```python
from build123d import *

# Parameters (mm, degrees)
EXTRUDE_1_DEPTH     = 20
SKETCH_9_W          = 35
SKETCH_9_H          = 3
EXTRUDE_2_DEPTH     = 5
SKETCH_10_W         = 3
SKETCH_10_H         = 35
EXTRUDE_3_DEPTH     = 5
SKETCH_11_R         = 8
CUT_EXTRUDE_4_DEPTH = 8
SKETCH_12_W         = 30
SKETCH_12_H         = 3
CUT_EXTRUDE_5_DEPTH = 18
SKETCH_13_W         = 30
SKETCH_13_H         = 17
CUT_EXTRUDE_6_DEPTH = 1
SKETCH_14_W         = 30
SKETCH_14_H         = 36
CUT_EXTRUDE_7_DEPTH = 1
SKETCH_15_R         = 1.5
CUT_EXTRUDE_8_DEPTH = 2
SKETCH_17_W         = 39.353314789
SKETCH_17_H         = 5.702998022
CUT_EXTRUDE_9_DEPTH = 8


with BuildPart() as part:
    # 草图1 → 凸台-拉伸1 (new body)
    with BuildSketch(Plane(origin=(0, 0, 0), x_dir=(0, 0, -1), z_dir=(1, 0, 0))):
        Polygon((0, 0), (0, 38), (3, 38), (3, 3), (38, 3), (38, 0), align=None)
    extrude(amount=EXTRUDE_1_DEPTH)

    # 草图9 → 凸台-拉伸2 (add)
    with BuildSketch(Plane(origin=(20, 0, 0), x_dir=(0, 0, -1), z_dir=(1, 0, 0))):
        Polygon((3, 38), (0, 38), (0, 0), (3, 0), (3, 3), align=None)
        with Locations((20.5, 1.5)):
            Rectangle(SKETCH_9_W, SKETCH_9_H)
    extrude(amount=EXTRUDE_2_DEPTH)

    # 草图10 → 凸台-拉伸3 (add)
    with BuildSketch(Plane.ZY):
        with Locations((-1.5, 20.5)):
            Rectangle(SKETCH_10_W, SKETCH_10_H)
        Polygon((0, 0), (0, 3), (-3, 3), (-38, 3), (-38, 0), align=None)
    extrude(amount=EXTRUDE_3_DEPTH)

    # 草图11 → 切除-拉伸4 (cut)
    with BuildSketch(Plane.XY):
        with Locations((10, 16)):
            Circle(SKETCH_11_R)
    extrude(amount=-CUT_EXTRUDE_4_DEPTH, mode=Mode.SUBTRACT)

    # 草图12 → 切除-拉伸5 (cut)
    with BuildSketch(Plane(origin=(0, 0, -38), x_dir=(-1, 0, 0), z_dir=(0, 0, -1))):
        with Locations((-10, 1.5)):
            Rectangle(SKETCH_12_W, SKETCH_12_H)
    extrude(amount=-CUT_EXTRUDE_5_DEPTH, mode=Mode.SUBTRACT)

    # 草图13 → 切除-拉伸6 (cut)
    with BuildSketch(Plane(origin=(0, 3, 0), x_dir=(1, 0, 0), z_dir=(0, 1, 0))):
        with Locations((10, 11.5)):
            Rectangle(SKETCH_13_W, SKETCH_13_H)
    extrude(amount=-CUT_EXTRUDE_6_DEPTH, mode=Mode.SUBTRACT)

    # 草图14 → 切除-拉伸7 (cut)
    with BuildSketch(Plane(origin=(0, 0, -3), x_dir=(-1, 0, 0), z_dir=(0, 0, -1))):
        with Locations((-10, 20)):
            Rectangle(SKETCH_14_W, SKETCH_14_H)
    extrude(amount=-CUT_EXTRUDE_7_DEPTH, mode=Mode.SUBTRACT)

    # 草图15 → 切除-拉伸8 (cut)
    with BuildSketch(Plane(origin=(0, 2, 0), x_dir=(1, 0, 0), z_dir=(0, 1, 0))):
        with Locations((20, 6)):
            Circle(SKETCH_15_R)
        with Locations((0, 6)):
            Circle(SKETCH_15_R)
        with Locations((0, 16)):
            Circle(SKETCH_15_R)
        with Locations((20, 16)):
            Circle(SKETCH_15_R)
    extrude(amount=-CUT_EXTRUDE_8_DEPTH, mode=Mode.SUBTRACT)

    # 草图17 → 切除-拉伸9 (cut)
    with BuildSketch(Plane(origin=(0, 38, 0), x_dir=(1, 0, 0), z_dir=(0, 1, 0))):
        with Locations((8.215909563, 1.4252762)):
            Rectangle(SKETCH_17_W, SKETCH_17_H)
    extrude(amount=-CUT_EXTRUDE_9_DEPTH, mode=Mode.SUBTRACT)


solid = part.part
```
Model file for the job. Use its own axes, mm. A direction names the side the tool comes from. Coordinates: 2 decimals unless noted, no trailing zeros. Loops run counter-clockwise (first coordinate to the right, second up) from the corner with the lowest first, then second, coordinate; pieces in that order, holes last. Notation, with made-up numbers: (1.5, -34) - (19.5, -34) arc R9 ccw to (19.5, -20) - close; hole circle Ø7 at (2.25, 28.5). An arc over 180 degrees is marked (long way). Write item = value, one per line. Start each with the question number.
Item 1: Saw through at C-C, the plane y = 16. List the corners of the cut face in (x, z), then the cut area to 3 significant figures.
Item 2: Wall check: probe 1 along X at (y, z) = (1.05, -6); probe 2 along Z at (x, y) = (20, 0.75); probe 3 along Y at (x, z) = (10, -0.45). Give the ranges that are in metal, low to high. Write a range as [from, to].
Item 3: Saw through at D-D, the plane x = 10. List the corners of the cut face in (y, z).
Item 4: Saw through at B-B, the plane x = 20. List the corners of the cut face in (y, z), then the cut area to 3 significant figures.
Item 5: Drop a flat-ended pin along its axis: pin 1 Ø10 at (x, z) = (22, -12) entering from +Y. Give the stop position or say it passes through.
Item 6: Saw through at A-A, the plane z = -6. List the corners of the cut face in (x, y), then the cut area to 3 significant figures.
Item 7: 3-axis set-ups, long thin cutter, end or side, ignore diameter. For faces 1 (the face through (10, 2, -11)), 2 (the face through (10, 1, -20)): which of +Z, -Z, +X, -X, +Y, -Y reach the whole face in a straight line?
Item 8: Pull direction X, two halves, no side cores. Call faces 3 (the face through (25, 10.6, -1.8)), 4 (the face through (18.5, 1.01, -6.07)), 5 (the face through (18.5, 1.01, -16.07)), 6 (the face through (14, 8, 0)): +X half, -X half, draft (parallel to the pull), parting line (faces both ways), or undercut.
Answers:
q1.outline = (-5, -2) - (2, -2) - (2, 0) - (-5, 0) - close; (18, -2) - (25, -2) - (25, 0) - (18, 0) - close
q1.area = 28.0 mm2
q2.probe_1 = [-5, -1.5], [1.5, 18.5], [21.5, 25]
q2.probe_2 = [-20, -17.5], [-14.5, -7.5], [-4.5, 0]
q2.probe_3 = [0, 8], [24, 30]
q3.outline = (0, -20) - (2, -20) - (2, -2) - (8, -2) - (8, 0) - (0, 0) - close; (24, -2) - (30, -2) - (30, 0) - (24, 0) - close
q4.outline = (0, -20) - (2, -20) - (2, -17.5) - (0, -17.5) - close; (0, -14.5) - (2, -14.5) - (2, -7.5) - (0, -7.5) - close; (0, -4.5) - (2, -4.5) - (2, -2) - (30, -2) - (30, 0) - (0, 0) - close
q4.area = 84.0 mm2
q5.pin_1 = 2
q6.outline = (-5, 0) - (-1.5, 0) - (-1.5, 2) - (-5, 2) - close; (1.5, 0) - (18.5, 0) - (18.5, 2) - (1.5, 2) - close; (21.5, 0) - (25, 0) - (25, 2) - (21.5, 2) - close
q6.area = 48.0 mm2
q7.face_1 = -Z, +X, -X, +Y
q7.face_2 = -Z, +X, -X, +Y, -Y
q8.face_3 = +X half
q8.face_4 = undercut
q8.face_5 = undercut
q8.face_6 = draft
